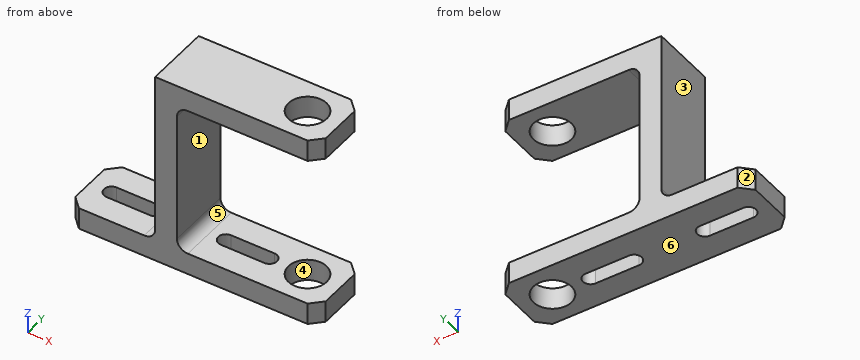
from build123d import *

# Parameters (mm, degrees)
BOSS_EXTRUDE1_DEPTH     = 30
SKETCH3_W               = 230
SKETCH3_H               = 60
SKETCH3_R               = 17.5
BOSS_EXTRUDE2_DEPTH     = 20
FILLET1_R               = 10
CHAMFER1_SIZE           = 10
SKETCH5_R               = 17.5
CUT_EXTRUDE1_DEPTH      = 1
CUT_EXTRUDE1_DEPTH_BACK = 181


with BuildPart() as part:
    # Sketch1 → Boss-Extrude1 (new body, symmetric)
    with BuildSketch(Plane(origin=(0, 0, 0), x_dir=(1, 0, 0), z_dir=(0, 1, 0))):
        Polygon((0, 160), (10, 160), (20, 160), (20, 20), (150, 20), (150, 0), (0, 0), align=None)
    extrude(amount=BOSS_EXTRUDE1_DEPTH, both=True)

    # Sketch3 → Boss-Extrude2 (add)
    with BuildSketch(Plane(origin=(0, 0, -160), x_dir=(-1, 0, 0), z_dir=(0, 0, -1))):
        with Locations((-35, 0)):
            Rectangle(SKETCH3_W, SKETCH3_H)
        with Locations((-120, 0)):
            Circle(SKETCH3_R, mode=Mode.SUBTRACT)
        with BuildLine():
            Line((60, -7), (20, -7))
            ThreePointArc((20, -7), (13, 0), (20, 7))
            Line((20, 7), (60, 7))
            ThreePointArc((60, 7), (67, 0), (60, -7))
        make_face(mode=Mode.SUBTRACT)
        with BuildLine():
            Line((-45, -7), (-85, -7))
            ThreePointArc((-85, -7), (-92, 0), (-85, 7))
            Line((-85, 7), (-45, 7))
            ThreePointArc((-45, 7), (-38, 0), (-45, -7))
        make_face(mode=Mode.SUBTRACT)
    extrude(amount=BOSS_EXTRUDE2_DEPTH)

    # Fillet1
    fillet1_edges = [part.edges().sort_by_distance(p)[0] for p in [
        (20, 0, -160),
        (20, 0, -20),
        (0, 0, -160),
    ]]
    fillet(fillet1_edges, radius=FILLET1_R)

    # Chamfer1
    chamfer1_edges = [part.edges().sort_by_distance(p)[0] for p in [
        (150, 30, -10),
        (150, 30, -170),
        (150, -30, -170),
        (-80, -30, -170),
        (-80, 30, -170),
        (150, -30, -10),
    ]]
    chamfer(chamfer1_edges, length=CHAMFER1_SIZE)

    # Sketch5 → Cut-Extrude1 (cut, two sides)
    with BuildSketch(Plane(origin=(0, 0, -180), x_dir=(-1, 0, 0), z_dir=(0, 0, -1))) as cut_extrude1_sk:
        with Locations((-120, 0)):
            Circle(SKETCH5_R)
    extrude(amount=CUT_EXTRUDE1_DEPTH, mode=Mode.SUBTRACT)
    extrude(cut_extrude1_sk.sketch, amount=-CUT_EXTRUDE1_DEPTH_BACK, mode=Mode.SUBTRACT)


solid = part.part
Design review of the part built by this model. Coordinates are the model's own, in mm. Face numbers are marked on the shaded views. A direction names the side the tool comes from. Give positions to 0.01 mm unless a question says otherwise; leave off trailing zeros. Order: outer loops, then holes, each group sorted by start corner. A loop starts at its lowest first (then second) coordinate and runs counter-clockwise, first axis right, second up. Notation, with made-up numbers: (-39, -21) - (-2, -21) arc R12 ccw to (-2, -3) - close; hole circle Ø4 at (63, 27). An arc over 180 degrees is marked (long way). Write item = value, one per line. Start each with the question number.
Q1. Mouldability with a two-part tool opening along Z and no side actions: class the marked faces 4, 5 and 6 as released by +Z, released by -Z, zero draft, split by the parting line, or undercut.
Q2. We need section A-A on y = 0. State how many separate pieces and enclosed holes the cut face has, plus the area to 3 significant figures.
Q3. We need section B-B on x = 120. State the section outline as (y, z) points, plus the area to 3 significant figures.
Q4. Tool access review of the marked faces 1, 2 and 3: name each direction out of +Z, -Z, +X, -X, +Y, -Y from which nothing blocks a thin tool from reaching the whole face with its end or side.
Q5. To check wall thickness, follow L1, parallel to Z at x = 139, y = -7; L2, parallel to Y at x = 120, z = -11; L3, parallel to Z at x = 50, y = -0.5. State the ranges of each line that lie inside material, in increasing order. Write a range as from..to.
Q6. We need section D-D on y = -23. State the section outline as (x, z) points, plus the area to 3 significant figures.
Q7. We need section C-C on x = 66. State the section outline as (y, z) points.
Q8. Clearance check with flat-ended pins moving along their axes: pin 1 Ø1.5 at (x, y) = (-29.5, 15.5) entering from +Z; pin 2 Ø4 at (y, z) = (-1.5, -71.5) entering from +X; pin 3 Ø2 at (y, z) = (-9.5, -75.5) entering from -X. State where each tip first meets the part, or that it passes through.
Working result:
q1.face_4 = zero draft
q1.face_5 = undercut
q1.face_6 = released by -Z
q2.separate_pieces = 5
q2.enclosed_holes = 0
q2.area = 6,900 mm²
q3.outline = (-30, -180) - (-17.5, -180) - (-17.5, -160) - (-30, -160) - close; (-30, -20) - (-17.5, -20) - (-17.5, 0) - (-30, 0) - close; (17.5, -180) - (30, -180) - (30, -160) - (17.5, -160) - close; (17.5, -20) - (30, -20) - (30, 0) - (17.5, 0) - close
q3.area = 1,000 mm²
q4.face_1 = +X, +Y, -Y
q4.face_2 = +Z, -Z, -X, +Y
q4.face_3 = +Z, -X, +Y, -Y
q5.L1 = -180..-160, -20..0
q5.L2 = -30..-17.5, 17.5..30
q5.L3 = -20..0
q6.outline = (-77, -180) - (147, -180) - (147, -160) - (30, -160) arc R10 cw to (20, -150) - (20, -30) arc R10 cw to (30, -20) - (147, -20) - (147, 0) - (0, 0) - (0, -150) arc R10 cw to (-10, -160) - (-77, -160) - close
q6.area = 10,300 mm²
q7.outline = (-30, -180) - (-7, -180) - (-7, -160) - (-30, -160) - close; (-30, -20) - (30, -20) - (30, 0) - (-30, 0) - close; (7, -180) - (30, -180) - (30, -160) - (7, -160) - close
q8.pin_1 = -160
q8.pin_2 = 20
q8.pin_3 = 0
